Geometry check sheet. Reference: drawing and pictorial views, mm from the part's lowest x, y, z. Give positions to 0.01 mm unless a question says otherwise; leave off trailing zeros. Loops run counter-clockwise (first coordinate to the right, second up) from the corner with the lowest first, then second, coordinate; pieces in that order, holes last. Notation, with made-up numbers: (12.5, -14.5) -> (52.5, -14.5) arc R18 cw to (52.5, -6.5) -> close; hole circle Ø6 at (76, 88). An arc over 180 degrees is marked (long way). One line per item, written item: value. Start each with the question number.
(1) Sectioned sample at B-B, the plane y = 18.5. Record the cut outline in (x, z).
(2) Scan lines: line 1 along Y through (x, z) = (111, 3.35); line 2 along X through (y, z) = (7.5, 1.2); line 3 along X through (y, z) = (20.5, 3.65). Record each from-to range of solid material in increasing order. Write a range as from..to.
(3) Gauge pin test, flat ends, axial feed: pin 1 Ø3 at (x, y) = (54, 18.5) entering from +Z; pin 2 Ø3 at (y, z) = (17, 4) entering from -X; pin 3 Ø1.5 at (x, z) = (59, 1) entering from -Y; pin 4 Ø1.5 at (y, z) = (26, 2) entering from +X. Record the tip position at first contact, or that the pin passes through.
(4) Sectioned sample at D-D, the plane x = 26. Record the cut outline in (y, z), then the cut area to 3 significant figures.
(5) Sectioned sample at A-A, the plane z = 3.3. State how many separate pieces and enclosed holes the cut face has, then the cut area to 3 significant figures.
(6) Sectioned sample at C-C, the plane y = 6.5. Record the cut outline in (x, z), then the cut area to 3 significant figures.
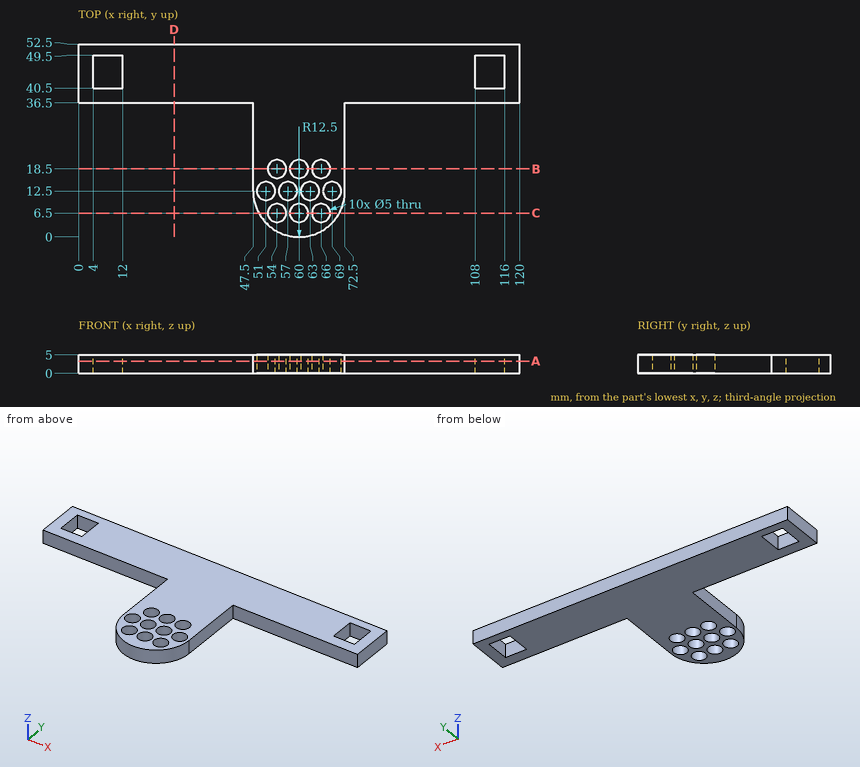
Calculated:
1. outline: (47.5, 0) -> (51.5, 0) -> (51.5, 5) -> (47.5, 5) -> close; (56.5, 0) -> (57.5, 0) -> (57.5, 5) -> (56.5, 5) -> close; (62.5, 0) -> (63.5, 0) -> (63.5, 5) -> (62.5, 5) -> close; (68.5, 0) -> (72.5, 0) -> (72.5, 5) -> (68.5, 5) -> close
2. line 1: y = 36.5..40.5, 49.5..52.5
2. line 2: x = 48.54..51.71, 56.29..57.71, 62.29..63.71, 68.29..71.46
2. line 3: x = 47.5..52.5, 55.5..58.5, 61.5..64.5, 67.5..72.5
3. pin 1: passes through
3. pin 2: stops at x = 47.5
3. pin 3: stops at y = 0
3. pin 4: stops at x = 72.5
4. outline: (36.5, 0) -> (52.5, 0) -> (52.5, 5) -> (36.5, 5) -> close
4. area: 80.0 mm2
5. separate pieces: 1
5. enclosed holes: 12
5. area: 2,430 mm2
6. outline: (49.03, 0) -> (51.5, 0) -> (51.5, 5) -> (49.03, 5) -> close; (56.5, 0) -> (57.5, 0) -> (57.5, 5) -> (56.5, 5) -> close; (62.5, 0) -> (63.5, 0) -> (63.5, 5) -> (62.5, 5) -> close; (68.5, 0) -> (70.97, 0) -> (70.97, 5) -> (68.5, 5) -> close
6. area: 34.7 mm2
